Input: part model. Units: mm. Frame: model coordinates. Face numbers are marked on the shaded views. Coordinates: 2 decimals unless noted, no trailing zeros. Write each loop counter-clockwise with the first axis right and the second up, starting at its lowest first coordinate (ties: lowest second). Pieces come first, ordered by that corner, then holes.
1) Pin query (flat end, axial travel): pin 1 Ø1.5 at (x, z) = (57.5, -50) entering from +Y; pin 2 Ø5 at (y, z) = (5.5, -5.5) entering from +X; pin 3 Ø5 at (x, z) = (124, -33) entering from -Y. Return the tip coordinate at first contact, or that it passes through.
2) Line query: L1, parallel to Z at x = 136.5, y = 6.5; L2, parallel to Z at x = 78, y = 9; L3, parallel to Z at x = 39.5, y = 0.25. Output: solid intervals per line, ascending.
3) Section query B-B (y = 9). Output: boundary loops of the cut face in (x, z), then the cut area to 3 significant figures.
4) Section query D-D (z = -68). Output: boundary loops of the cut face in (x, y).
5) Section query A-A (x = 26.5). Output: boundary loops of the cut face in (y, z), then the cut area to 3 significant figures.
6) Draft query along Z for the marked faces 1, 2 and 3. Return one class per face: pulls with the +Z half, pulls with the -Z half, needs draft (parallel to the pull), parting line crosses it, or undercut.
7) Section query C-C (z = -11.5). Output: boundary loops of the cut face in (x, y).
from build123d import *

# Parameters (mm, degrees)
BOSS_EXTRUDE1_DEPTH = 14
BOSS_EXTRUDE2_DEPTH = 1
BOSS_EXTRUDE3_DEPTH = 155.94
SKETCH1_5_W         = 14.94
SKETCH1_5_H         = 3
CUT_EXTRUDE1_DEPTH  = 10
BOSS_EXTRUDE4_DEPTH = 7.83
FILLET1_R           = 3
BOSS_EXTRUDE5_DEPTH = 7
SKETCH5_W           = 8.1
SKETCH5_H           = 5
CUT_EXTRUDE2_DEPTH  = 5


with BuildPart() as part:
    # Sketch1 → Boss-Extrude1 (new body)
    with BuildSketch(Plane(origin=(0, 0, 0), x_dir=(1, 0, 0), z_dir=(0, 1, 0))):
        Polygon((152.94, 117.29), (152.94, 114.29), (0, 114.29), (0, 0), (138, 0), (138, -3), (-3, -3), (-3, 117.29), align=None)
    extrude(amount=BOSS_EXTRUDE1_DEPTH)

    # Sketch1<3> → Boss-Extrude2 (add)
    with BuildSketch(Plane(origin=(0, 0, 0), x_dir=(1, 0, 0), z_dir=(0, 1, 0))):
        Polygon((138, 38.29), (138, 0), (0, 0), (0, 114.29), (152.94, 114.29), (152.94, 76.49), (143.44, 76.49), (143.44, 57.19), (148.2, 57.19), (148.2, 38.29), align=None)
        Polygon((152.94, 117.29), (152.94, 114.29), (0, 114.29), (0, 0), (138, 0), (138, -3), (-3, -3), (-3, 117.29), align=None)
    extrude(amount=-BOSS_EXTRUDE2_DEPTH)

    # Sketch2 → Boss-Extrude3 (add)
    with BuildSketch(Plane(origin=(152.94, 0, 0), x_dir=(0, 0, -1), z_dir=(1, 0, 0))):
        Polygon((117.29, 0), (117.29, -7.30413177), (-3, -1), (-3, 0), align=None)
    extrude(amount=-BOSS_EXTRUDE3_DEPTH)

    # Sketch1<5> → Cut-Extrude1 (cut)
    with BuildSketch(Plane(origin=(0, 0, 0), x_dir=(1, 0, 0), z_dir=(0, 1, 0))):
        with Locations((145.47, -1.5)):
            Rectangle(SKETCH1_5_W, SKETCH1_5_H)
        Polygon((138, 0), (152.94, 0), (152.94, 76.49), (143.44, 76.49), (143.44, 57.19), (148.2, 57.19), (148.2, 38.29), (138, 38.29), align=None)
    extrude(amount=-CUT_EXTRUDE1_DEPTH, mode=Mode.SUBTRACT)

    # Sketch3 → Boss-Extrude4 (add)
    with BuildSketch(Plane(origin=(138, 0, 0), x_dir=(0, 0, -1), z_dir=(1, 0, 0))):
        Polygon((19.09, -2.157687844), (19.09, 0), (0, 0), (0, 14), (-3, 14), (-3, -1), align=None)
    extrude(amount=BOSS_EXTRUDE4_DEPTH)

    # Fillet1
    fillet1_edges = [part.edges().sort_by_distance(p)[0] for p in [
        (-3, 6.5, 3),
        (-3, 3.347934115, -117.29),
    ]]
    fillet(fillet1_edges, radius=FILLET1_R)

    # Sketch4 → Boss-Extrude5 (add)
    with BuildSketch(Plane(origin=(0, 0, 0), x_dir=(1, 0, 0), z_dir=(0, 1, 0))):
        Polygon((0, 0), (145.83, 0), (145.83, 19.09), (138, 19.09), (138, 38.29), (148.2, 38.29), (148.2, 57.19), (143.44, 57.19), (143.44, 76.49), (152.94, 76.49), (152.94, 114.29), (0, 114.29), align=None)
        Polygon((150.94, 112.29), (2, 112.29), (2, 2), (143.83, 2), (143.83, 17.09), (136, 17.09), (136, 40.29), (146.2, 40.29), (146.2, 55.19), (141.44, 55.19), (141.44, 78.49), (150.94, 78.49), align=None, mode=Mode.SUBTRACT)
    extrude(amount=BOSS_EXTRUDE5_DEPTH)

    # Sketch5 → Cut-Extrude2 (cut)
    with BuildSketch(Plane(origin=(2, 0, 0), x_dir=(0, 0, -1), z_dir=(1, 0, 0))):
        with Locations((83.74, 2.5)):
            Rectangle(SKETCH5_W, SKETCH5_H)
    extrude(amount=-CUT_EXTRUDE2_DEPTH, mode=Mode.SUBTRACT)


solid = part.part
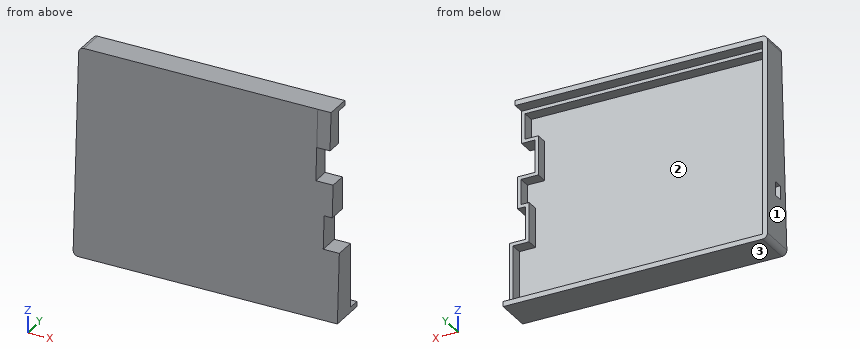
Answer:
1. pin 1: stops at y = 0
1. pin 2: stops at x = 145.83
1. pin 3: stops at y = -3.02
2. L1: z = -117.29 to -112.29, -40.29 to -17.09, -2 to 3
2. L2: z = -117.29 to -114.29, 0 to 3
2. L3: z = -117.29 to -112.29, -2 to 3
3. outline: (-3, -114.29) arc R3 ccw to (0, -117.29) - (152.94, -117.29) - (152.94, -114.29) - (0, -114.29) - (0, 0) - (145.83, 0) - (145.83, 3) - (0, 3) arc R3 ccw to (-3, 0) - close
3. area: 1,250 mm2
4. outline: (-3, -4.72) - (143.44, -4.72) - (143.44, 7) - (141.44, 7) - (141.44, 0) - (2, 0) - (2, 7) - (0, 7) - (0, 14) - (-3, 14) - close
5. outline: (-7.3, -117.29) - (14, -117.29) - (14, -114.29) - (7, -114.29) - (7, -112.29) - (0, -112.29) - (0, -2) - (7, -2) - (7, 0) - (14, 0) - (14, 3) - (-1, 3) - close
5. area: 611 mm2
6. face 1: needs draft
6. face 2: undercut
6. face 3: pulls with the -Z half
7. outline: (-3, -1.76) - (145.83, -1.76) - (145.83, 7) - (143.83, 7) - (143.83, 0) - (2, 0) - (2, 7) - (0, 7) - (0, 14) - (-3, 14) - close
